Verification items for this drawing (mm, ordinates from the low corner). Round coordinates to 2 decimals unless told otherwise and drop trailing zeros. Order: outer loops, then holes, each group sorted by start corner. A loop starts at its lowest first (then second) coordinate and runs counter-clockwise, first axis right, second up. Notation, with made-up numbers: M 31.5,64.25 L 37.5,64.25 A7 cw 37.5,76.25 Z; hole C 73.5,-2 d3. An arc over 180 degrees is marked long. One line per item, written item: value. Start each with the question number.
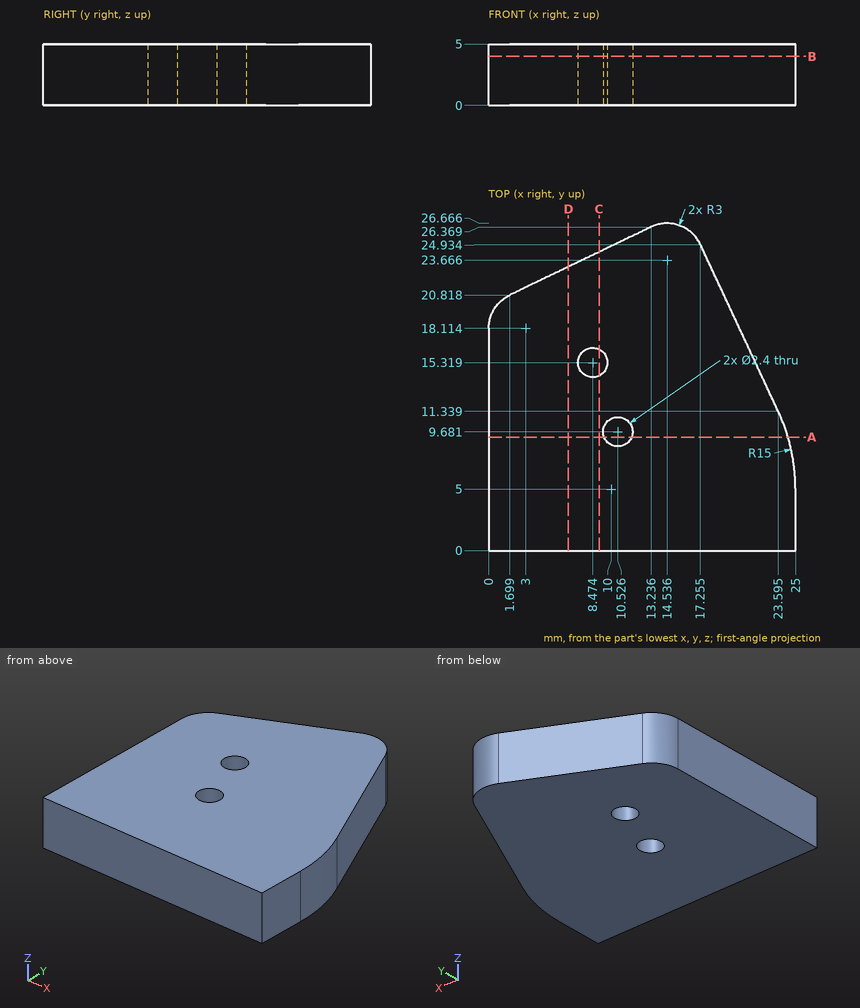
1. Section check C-C (x = 9). Record the cut outline in (y, z).
2. Depth check by flat-ended pin: pin 1 (1 mm diameter, centred on x = 9, z = 1.5, fed in from +Y); pin 2 (3 mm diameter, centred on y = 19.5, z = 2.5, fed in from +X); pin 3 (1 mm diameter, centred on x = 19.5, z = 1.5, fed in from +Y) (1 decimal). Enter the tip coordinate at first touch or a pass-through.
3. Section check A-A (y = 9.25). Record the cut outline in (x, z) (1 decimal), and give its area (3 significant figures).
4. Section check B-B (z = 4). Record the cut outline in (x, y) (1 decimal), and give its area (3 significant figures).
5. Section check D-D (x = 6.5). Record the cut outline in (y, z), and give its area (3 significant figures).
6. Scan lines: line 1 along X through (y, z) = (10, 0.7); line 2 along Y through (x, z) = (2.5, 2.7); line 3 along X through (y, z) = (17.25, 4.4). Record each from-to range of solid material in increasing order.
Geometry check:
1. outline: M 0,0 L 14.24,0 L 14.24,5 L 0,5 Z; M 16.4,0 L 24.33,0 L 24.33,5 L 16.4,5 Z
2. pin 1: stops at y = 24.57
2. pin 2: stops at x = 20.49
2. pin 3: stops at y = 21.2
3. outline: M 0,0 L 9.4,0 L 9.4,5 L 0,5 Z; M 11.6,0 L 24.4,0 L 24.4,5 L 11.6,5 Z
3. area: 111 mm²
4. outline: M 0,0 L 25,0 L 25,5 A15 ccw 23.6,11.3 L 17.3,24.9 A3 ccw 13.2,26.4 L 1.7,20.8 A3 ccw 0,18.1 Z; hole C 8.5,15.3 d2.4; hole C 10.5,9.7 d2.4
4. area: 531 mm²
5. outline: M 0,0 L 23.13,0 L 23.13,5 L 0,5 Z
5. area: 116 mm²
6. line 1: x = 0 to 9.37, 11.68 to 24.14
6. line 2: y = 0 to 21.2
6. line 3: x = 0 to 20.84
